from build123d import *

# Parameters (mm, degrees)
BOSS_EXTRU_1_DEPTH      = 6
ESQUISSE2_R             = 1.5
ENL_V_MAT_EXTRU_1_DEPTH = 75.67261881
ESQUISSE3_R             = 3
ENL_V_MAT_EXTRU_2_DEPTH = 3


with BuildPart() as part:
    # Esquisse1 → Boss.-Extru.1 (new body)
    with BuildSketch(Plane.XY):
        Polygon((0, -32), (-17, -32), (-17, -38), (-47, -38), (-47, -32), (-64, -32), (-64, 0), (0, 0), align=None)
    extrude(amount=BOSS_EXTRU_1_DEPTH)

    # Esquisse2 → Enlèv. mat.-Extru.1 (cut, through all)
    with BuildSketch(Plane(origin=(0, 0, 0), x_dir=(-1, 0, 0), z_dir=(0, 0, -1))):
        with Locations((14, -4)):
            Circle(ESQUISSE2_R)
        with Locations((4, -24)):
            Circle(ESQUISSE2_R)
        with Locations((24, -24)):
            Circle(ESQUISSE2_R)
        with Locations(Location((40, -24, 0), (0, 0, 180))):
            Circle(ESQUISSE2_R)
        with Locations(Location((60, -24, 0), (0, 0, 180))):
            Circle(ESQUISSE2_R)
        with Locations(Location((50, -4, 0), (0, 0, 180))):
            Circle(ESQUISSE2_R)
    extrude(amount=-ENL_V_MAT_EXTRU_1_DEPTH, mode=Mode.SUBTRACT)

    # Esquisse3 → Enlèv. mat.-Extru.2 (cut)
    with BuildSketch(Plane(origin=(0, 0, 0), x_dir=(-1, 0, 0), z_dir=(0, 0, -1))):
        with Locations((14, -4)):
            Circle(ESQUISSE3_R)
        with Locations((4, -24)):
            Circle(ESQUISSE3_R)
        with Locations((24, -24)):
            Circle(ESQUISSE3_R)
        with Locations((40, -24)):
            Circle(ESQUISSE3_R)
        with Locations((60, -24)):
            Circle(ESQUISSE3_R)
        with Locations((50, -4)):
            Circle(ESQUISSE3_R)
    extrude(amount=-ENL_V_MAT_EXTRU_2_DEPTH, mode=Mode.SUBTRACT)


solid = part.part
Check sheet for the modelled part. Datum: model origin and axes. Units: mm. A direction names the side the tool comes from. Round coordinates to 2 decimals unless told otherwise and drop trailing zeros. Loops run counter-clockwise (first coordinate to the right, second up) from the corner with the lowest first, then second, coordinate; pieces in that order, holes last. Notation, with made-up numbers: M 18.25,23 L 64.25,23 A17 cw 64.25,48 Z; hole C -34,75 d7. An arc over 180 degrees is marked long. One line per question, with ' | ' between items. Start each with the question number.
Item 1: Section check C-C (z = 1.65). Record the boundary of the cut face in (x, y).
Item 2: Section check A-A (y = -4). Record the boundary of the cut face in (x, z).
Item 3: Scan lines: probe 1 along Y at (x, z) = (-50, 1.65); probe 2 along Y at (x, z) = (-40, 1.3); probe 3 along X at (y, z) = (-24.5, 1.6). Record each from-to range of solid material in increasing order.
Item 4: Section check B-B (x = -60). Record the boundary of the cut face in (y, z).
Item 5: Set-up check for faces 5 (the face through (-17, -35, 3)), 6 (the face through (-32, -19, 0)), 7 (the face through (-21, -24, 1)): record each of +Z, -Z, +X, -X, +Y, -Y from which the full face is reachable in a straight line by a thin tool's end or side.
Item 6: Section check D-D (x = -24). Record the boundary of the cut face in (y, z), and give its area (3 significant figures).
Item 7: Release check for a two-part mould opening along X. For faces 1 (the face through (-47, -35, 3)), 2 (the face through (-41.3, -25.3, 3)), 3 (the face through (-32, 0, 3)), 4 (the face through (0, -16, 3)) record: released by +X, released by -X, zero draft, split by the parting line, or undercut.
Item 8: Gauge pin test, flat ends, axial feed: pin 1 Ø3.5 at (x, y) = (-24, -24) entering from +Z; pin 2 Ø2.5 at (x, y) = (-50, -4) entering from +Z; pin 3 Ø3 at (x, y) = (-41, -24.5) entering from -Z. Record the tip position at first contact, or that the pin passes through.
Worked out:
1) outline: M -64,-32 L -47,-32 L -47,-38 L -17,-38 L -17,-32 L 0,-32 L 0,0 L -64,0 Z; hole C -60,-24 d6; hole C -50,-4 d6; hole C -40,-24 d6; hole C -24,-24 d6; hole C -14,-4 d6; hole C -4,-24 d6
2) outline: M -64,0 L -53,0 L -53,3 L -51.5,3 L -51.5,6 L -64,6 Z; M -48.5,3 L -47,3 L -47,0 L -17,0 L -17,3 L -15.5,3 L -15.5,6 L -48.5,6 Z; M -12.5,3 L -11,3 L -11,0 L 0,0 L 0,6 L -12.5,6 Z
3) probe 1: -32 to -7, -1 to 0 | probe 2: -38 to -27, -21 to 0 | probe 3: -64 to -62.96, -57.04 to -42.96, -37.04 to -26.96, -21.04 to -6.96, -1.04 to 0
4) outline: M -32,0 L -27,0 L -27,3 L -25.5,3 L -25.5,6 L -32,6 Z; M -22.5,3 L -21,3 L -21,0 L 0,0 L 0,6 L -22.5,6 Z
5) face 5: +Z, -Z, +X, -Y | face 6: -Z, +X, -X, +Y, -Y | face 7: -Z
6) outline: M -38,0 L -27,0 L -27,3 L -25.5,3 L -25.5,6 L -38,6 Z; M -22.5,3 L -21,3 L -21,0 L 0,0 L 0,6 L -22.5,6 Z | area: 201 mm^2
7) face 1: released by -X | face 2: undercut | face 3: zero draft | face 4: released by +X
8) pin 1: z = 6 | pin 2: through | pin 3: z = 3
